from build123d import *

# Parameters (mm, degrees)
SKETCH1_R                                       = 2
SKETCH1_R_2                                     = 5
BOSS_EXTRUDE1_DEPTH                             = 10
CSK_FOR_M3_FLAT_HEAD_MACHINE_SCREW1_D           = 3.4
CSK_FOR_M3_FLAT_HEAD_MACHINE_SCREW1_CSINK_D     = 6.3
CSK_FOR_M3_FLAT_HEAD_MACHINE_SCREW1_CSINK_ANGLE = 90
BOSS_EXTRUDE2_DEPTH                             = 5
F_3_0MM_DOWEL_HOLE1_D                           = 3.5


with BuildPart() as part:
    # Sketch1 → Boss-Extrude1 (new body)
    with BuildSketch(Plane(origin=(0, 0, 0), x_dir=(0, 0, -1), z_dir=(1, 0, 0))):
        with BuildLine():
            Line((30, -15), (20, -15))
            Line((20, -15), (20, 0))
            ThreePointArc((20, 0), (0, 20), (-20, 0))
            Line((-20, 0), (-20, -15))
            Line((-20, -15), (-20, -20))
            Line((-20, -20), (-15.856579477, -20))
            Line((-15.856579477, -20), (9.951007048, -20))
            Line((9.951007048, -20), (17.640087429, -20))
            Line((17.640087429, -20), (30, -20))
            Line((30, -20), (30, -15))
        make_face()
        with Locations((-9.526279442, -5.5)):
            Circle(SKETCH1_R, mode=Mode.SUBTRACT)
        with Locations((0, -11)):
            Circle(SKETCH1_R, mode=Mode.SUBTRACT)
        with Locations((9.526279442, -5.5)):
            Circle(SKETCH1_R, mode=Mode.SUBTRACT)
        with Locations((-9.526279442, 5.5)):
            Circle(SKETCH1_R, mode=Mode.SUBTRACT)
        Circle(SKETCH1_R_2, mode=Mode.SUBTRACT)
        with Locations((9.526279442, 5.5)):
            Circle(SKETCH1_R, mode=Mode.SUBTRACT)
        with Locations((0, 11)):
            Circle(SKETCH1_R, mode=Mode.SUBTRACT)
    extrude(amount=BOSS_EXTRUDE1_DEPTH)

    # CSK for M3 Flat Head Machine Screw1 (through all)
    with Locations(Plane.ZY):
        with Locations((0, 11), (9.526279442, 5.5), (9.526279442, -5.5), (0, -11), (-9.526279442, -5.5), (-9.526279442, 5.5)):
            CounterSinkHole(CSK_FOR_M3_FLAT_HEAD_MACHINE_SCREW1_D / 2, CSK_FOR_M3_FLAT_HEAD_MACHINE_SCREW1_CSINK_D / 2, counter_sink_angle=CSK_FOR_M3_FLAT_HEAD_MACHINE_SCREW1_CSINK_ANGLE)

    # Sketch6 → Boss-Extrude2 (add)
    with BuildSketch(Plane.XZ.offset(20)):
        Polygon((0, 20), (-10, 20), (-10, 10), (0, 10), (10, 10), (10, 20), align=None)
    extrude(amount=-BOSS_EXTRUDE2_DEPTH)

    # Ø3.0mm Dowel Hole1 (through all)
    with Locations(Plane(origin=(5, -15, -25), x_dir=(0, 0, 1), z_dir=(0, 1, 0))):
        with Locations((0, 0), (40, -10)):
            Hole(F_3_0MM_DOWEL_HOLE1_D / 2)


solid = part.part
Could you check a few things on this model? Use its own coordinates, in mm. A direction names the side the tool comes from. Give positions to 0.01 mm unless a question says otherwise; leave off trailing zeros. Order: outer loops, then holes, each group sorted by start corner. A loop starts at its lowest first (then second) coordinate and runs counter-clockwise, first axis right, second up. Notation, with made-up numbers: (83, 57.25) -> (140, 57.25) arc R11 cw to (140, 64.25) -> close; hole circle Ø11 at (70.25, 72). An arc over 180 degrees is marked (long way). Answer in a Markdown table with one row per item. Add a question column.
Item 1: Imagine slicing it at C-C (y = 1). List the corners of the cut face in (x, z) for me.
Item 2: Please list where these lines run through material, in increasing order: probe 1 along Z at (x, y) = (5.25, -5.5); probe 2 along Y at (x, z) = (7.25, 0); probe 3 along X at (y, z) = (-16, 15).
Item 3: I'm going to push flat-ended pins straight in: P1, Ø5, axis at x = 7, z = -23, coming from the +Y side; P2, Ø1.5, axis at x = 7, y = 9.5, coming from the -Z side; P3, Ø5, axis at y = -5.5, z = -9.53, coming from the -X side. Where does each tip first touch, or does it pass through?
Item 4: Imagine slicing it at A-A (x = 5). Count the separate pieces of the cut face and the enclosed holes in it, and give its area (3 significant figures).
Item 5: Imagine slicing it at D-D (z = -16). List the corners of the cut face in (x, y) for me, and give its area (3 significant figures).
Item 6: We'd pull the mould along Z, two halves only. Please class faces 4 (the cylindrical face through (-5.67, -17.535, 13.383)), 5 (the flat face through (0, -4, -5)), 6 (the flat face through (5, -8, -20)): pulls with the +Z half, pulls with the -Z half, needs draft (parallel to the pull), parting line crosses it, or undercut.
Item 7: For faces 1 (the flat face through (-5, -15, 13)), 2 (the flat face through (5, -18, -30)), 3 (the flat face through (3, -15, -25)), which set-ups out of +Z, -Z, +X, -X, +Y, -Y let a thin tool reach every point of the face, with its end or its side?
Item 8: Imagine slicing it at B-B (z = -25). List the corners of the cut face in (x, y) for me.
Result:
| question | item | result |
|---|---|---|
| 1 | outline | (0, -19.97) -> (10, -19.97) -> (10, -4.9) -> (0, -4.9) -> close; (0, 4.9) -> (10, 4.9) -> (10, 19.97) -> (0, 19.97) -> close |
| 2 | probe 1 | -20 to -11.53, -7.53 to 7.53, 11.53 to 20 |
| 2 | probe 2 | -20 to -13, -9 to -5, 5 to 9, 13 to 20 |
| 2 | probe 3 | -10 to -6.75, -3.25 to 10 |
| 3 | P1 | y = -15 |
| 3 | P2 | z = -17.98 |
| 3 | P3 | x = 0.65 |
| 4 | separate pieces | 2 |
| 4 | enclosed holes | 7 |
| 4 | area | 1,310 mm2 |
| 5 | outline | (0, -20) -> (10, -20) -> (10, 12) -> (0, 12) -> close |
| 5 | area | 320 mm2 |
| 6 | face 4 | undercut |
| 6 | face 5 | needs draft |
| 6 | face 6 | pulls with the -Z half |
| 7 | face 1 | +Z, -Z, -X, +Y |
| 7 | face 2 | -Z, +X, -X, +Y, -Y |
| 7 | face 3 | -Z, +X, -X, +Y |
| 8 | outline | (0, -20) -> (3.25, -20) -> (3.25, -15) -> (0, -15) -> close; (6.75, -20) -> (10, -20) -> (10, -15) -> (6.75, -15) -> close |
